Drawing for the job (mm, zero at the part's lowest x, y, z). Coordinates: 2 decimals unless noted, no trailing zeros. Write each loop counter-clockwise with the first axis right and the second up, starting at its lowest first coordinate (ties: lowest second). Pieces come first, ordered by that corner, then holes. Notation, with made-up numbers: (-23.5, 54.5) -> (-19.5, 54.5) arc R3 cw to (-19.5, 58.5) -> close; hole circle Ø10 at (-13.5, 82.25). An arc over 180 degrees is marked (long way). Write item = value, one per line. Start each with the question number.
Q1. Band-saw the part on C-C, the plane z = 0.95. List the corners of the cut face in (x, y) (1 decimal).
Q2. Band-saw the part on A-A, the plane y = 11.75. List the corners of the cut face in (x, z) (1 decimal).
Q3. Probe line 1 (Y direction, x = 53, z = 2.65); line 2 (Y direction, x = 27.5, z = 2.6) (1 decimal); line 3 (Y direction, x = 45, z = 2.05). List the from-to ranges inside material, lowest first.
Q4. Pull direction Y, two halves, no side cores. Call the marked faces 1, 2, 3 and 4: released by +Y, released by -Y, zero draft, split by the parting line, or undercut.
Q5. Pin check, flat tip, straight feed: P1, Ø4, axis at x = 53.29, y = 12.7, coming from the -Z side (3 decimals). Stop position of the tip, or through.
Q6. Band-saw the part on B-B, the plane x = 7.5. List the corners of the cut face in (y, z) (1 decimal).
Q7. Band-saw the part on D-D, the plane x = 42.5. List the corners of the cut face in (y, z) (1 decimal).
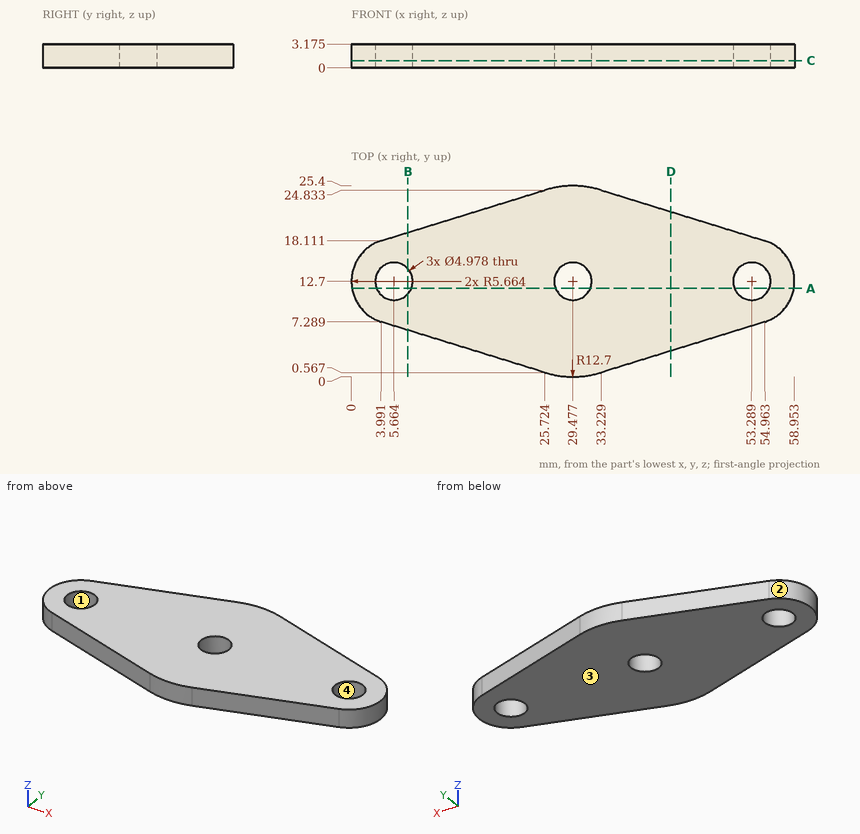
Ans:
q1.outline = (4, 7.3) -> (25.7, 0.6) arc R12.7 ccw to (33.2, 0.6) -> (55, 7.3) arc R5.7 ccw to (55, 18.1) -> (33.2, 24.8) arc R12.7 ccw to (25.7, 24.8) -> (4, 18.1) arc R5.7 ccw to start; hole circle Ø5 at (5.7, 12.7); hole circle Ø5 at (29.5, 12.7); hole circle Ø5 at (53.3, 12.7)
q2.outline = (0.1, 0) -> (3.4, 0) -> (3.4, 3.2) -> (0.1, 3.2) -> close; (8, 0) -> (27.2, 0) -> (27.2, 3.2) -> (8, 3.2) -> close; (31.8, 0) -> (51, 0) -> (51, 3.2) -> (31.8, 3.2) -> close; (55.6, 0) -> (58.9, 0) -> (58.9, 3.2) -> (55.6, 3.2) -> close
q3.line_1 = 6.68 to 10.23, 15.17 to 18.72
q3.line_2 = 0.2 to 11.2, 14.2 to 25.2
q3.line_3 = 4.21 to 21.19
q4.face_1 = undercut
q4.face_2 = split by the parting line
q4.face_3 = zero draft
q4.face_4 = undercut
q5.P1 = through
q6.outline = (6.2, 0) -> (11, 0) -> (11, 3.2) -> (6.2, 3.2) -> close; (14.4, 0) -> (19.2, 0) -> (19.2, 3.2) -> (14.4, 3.2) -> close
q7.outline = (3.4, 0) -> (22, 0) -> (22, 3.2) -> (3.4, 3.2) -> close
